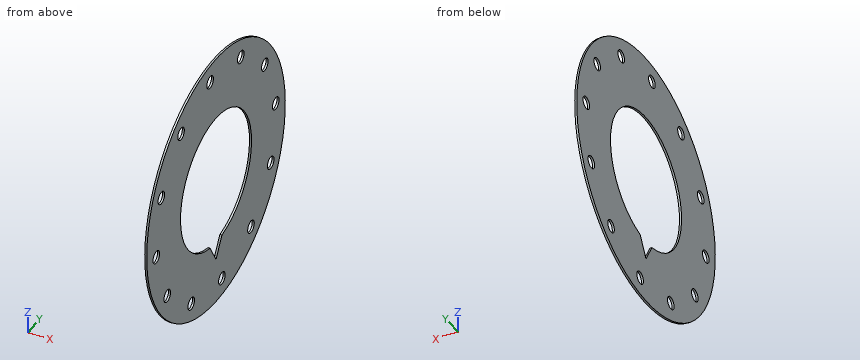
Autodesk Inventor part; units mm, degrees
ref_plane "SHAFT_MOUNTING_PLANE" through (9.525, 0, 0) normal (1, 0, 0) x (0, 1, 0)
ref_plane "UCSBasePlConstraintOrigin: YZ Plane" through (0, 0, 0) normal (0, 0, -1) x (0, 1, 0)
ref_plane "UCSBasePlConstraintOrigin: XZ Plane" through (0, 0, 0) normal (0, 1, 0) x (1, 0, 0)
ref_plane "BASE_PLATE_FACE" through (9.525, 0, 0) normal (1, 0, 0) x (0, 1, 0)
sketch "BASE_PLATE_SKETCH" plane through (9.525, 0, 0) normal (1, 0, 0) x (0, 0, -1)
  circle A0 centre (0, 0) radius 536.575 construction
  circle A1 centre (0, 0) radius 317.5
  line L0 (0, 536.575) -> (0, 536.575) construction
  circle A2 centre (0, 0) radius 619.125
  line L1 (0, 0) -> (-52.5935, -533.9912) construction
  line L2 (0, 0) -> (52.5935, -533.9912) construction
  line L3 (313.0592, 52.9167) -> (404.7136, 0)
  line L4 (404.7136, 0) -> (313.0592, -52.9167)
  line L5 (313.0592, -52.9167) -> (313.0592, 52.9167)
  line L6 (0, 0) -> (0, 536.575) construction
  line L7 (0, 0) -> (267.5578, 465.1081) construction
  point P0 (-619.125, 0)
  point P1 (619.125, 0)
  point P2 (0, 619.125)
  point P3 (0, -619.125)
  point P4 (0, 619.125)
  point P5 (619.125, 0)
  point P6 (0, -619.125)
  point P7 (-619.125, 0)
  point P8 (343.6107, 0)
  point P9 (313.0592, 0)
  point P10 (313.0592, -52.9167)
  dimension "GapSize" = 9.525
  dimension "SeamGap" = 0.0051
  dimension "Thickness" = 9.525
  dimension "BendRadius" = 9.525
  dimension "MinimumRemnant" = 19.05
  dimension "BendReliefDepth" = 4.7625
  dimension "BendReliefWidth" = 9.525
  dimension "CornerReliefSize" = 38.1
  dimension "JacobiRadiusSize" = 9.525
  dimension "TransitionRadius" = 9.525
  dimension "TEMPLATE_CENTER_HOLE_DIA" = 635
  dimension "NUMBER_OF_HOLES_IN_BOLT_PLATE" = 12
  dimension "BOLT_CIRCLE_DIA" = 1073.15
  dimension "TEMPLATE_DIA" = 1238.25
  dimension "PARENT_HOLE_ANG_L" = 5.625
  dimension "PARENT_HOLE_ANG_R" = 5.625
  dimension "NOTCH_LEG" = 105.8333
  dimension "d297" = 105.8333
  dimension "LEADER_PLACE_A_ANG" = 29.91
extrude "BASE_PLATE_BODY" add sketch "BASE_PLATE_SKETCH" against normal up to surface (9.525 mm away) contours A1 L3 L4 | A2
ref_plane "SHAFT_MOUNTING_PLANE" through (9.525, 0, 0) normal (1, 0, 0) x (0, 1, 0)
hole "PARENT_HOLE" at (9.525, -533.9912, -52.5935) direction (-1, 0, 0) diameter 58.7375 depth 9.525 tip angle 118
pattern_circular "BOLT_HOLES" count 12 over 360 about axis through (-10, 0, 0) along (1, 0, 0) of "PARENT_HOLE"
ref_plane "DimPlaneRight" through (0, 0, -619.125) normal (0, 0, 1) x (1, 0, 0)
ref_plane "DimPlaneLeft" through (0, 0, 619.125) normal (0, 0, 1) x (1, 0, 0)
ref_plane "DimPlaneTop" through (0, 619.125, 0) normal (0, 1, 0) x (-1, 0, 0)
ref_plane "DimPlaneBtm" through (0, -619.125, 0) normal (0, 1, 0) x (-1, 0, 0)
ref_plane "PLPointBngPltCenterHoleDia" through (0, 0, 0) normal (0, -0.866, 0.5) x (1, 0, 0)
extrude "V NOTCH CUT" cut sketch "BASE_PLATE_SKETCH" against normal through all contours A1 L3 L4
equation "\"BOLT_CIRCLE_DIA\" = INPUT_BOLT_CIRCLE_DIAMETER"
equation "\"INPUT_TEMPLATE_DIAMETER\" = 1238.25"
equation "\"INPUT_BOLT_HOLE_SIZE\" = 58.7375"
equation "\"INPUT_BOLT_CIRCLE_DIAMETER\" = 1073.15"
equation "\"INPUT_PARENT_HOLE_ANG_OFF_90_270\" = 5.625deg"
equation "\"SHAFT_B_DIST_AK_BOTTOM\" = 933.5008"
equation "\"SHAFT_B_DIST_AF_BOTTOM\" = 901.7"
equation "\"SHAFT_B_Thickness\" = 7.9502"
equation "\"INPUT_CENTER_HOLE_DIAMETER\" = 635"
equation "\"LEADER_PLACE_A\" = 68.5deg"
equation "\"TEMPLATE_RAD\" = 619.125"
properties part number "25-00000E_TEMPLATE_TOP" material "A572 GRADE 65"
Here's how the part is built. I have some questions about the finished solid (model axes, mm). Coordinates: 2 decimals unless noted, no trailing zeros. Write each loop counter-clockwise with the first axis right and the second up, starting at its lowest first coordinate (ties: lowest second). Pieces come first, ordered by that corner, then holes. Notation, with made-up numbers: (39.25, 84) - (60.25, 84) arc R20 cw to (60.25, 108) - close; hole circle Ø6 at (57, 43). An arc over 180 degrees is marked (long way). Use one line per item in the form item = value.
1) Suppose I cut it at C-C, the plane x = 6.25. Give the number of separate pieces and of enclosed holes in the cut face, plus the area to 3 significant figures.
Solved:
separate_pieces = 1
enclosed_holes = 13
area = 850,000 mm2
2) I need wall thicknesses on line 1 (Z direction, x = 2.5, y = -247); line 2 (Z direction, x = 6, y = 221.5); line 3 (Y direction, x = 3.75, z = 0) (3 decimals). Which ranges of each line are inside material? Lowest first, please.
Solved:
line_1 = -567.72 to -503.23, -474.27 to -199.49, 199.49 to 567.72
line_2 = -578.15 to -227.47, 227.47 to 459.38, 518.12 to 578.15
line_3 = -619.125 to -317.5, 317.5 to 619.125
3) Suppose I cut it at B-B, the plane z = 298. Write out the boundary of the cut face in (x, y) (3 decimals).
Solved:
outline = (0, -542.689) - (9.525, -542.689) - (9.525, -109.555) - (0, -109.555) - close; (0, 109.555) - (9.525, 109.555) - (9.525, 410.638) - (0, 410.638) - close; (0, 461.668) - (9.525, 461.668) - (9.525, 542.689) - (0, 542.689) - close
4) Suppose I cut it at D-D, the plane z = -210.5. Write out the boundary of the cut face in (x, y) (3 decimals).
Solved:
outline = (0, -582.242) - (9.525, -582.242) - (9.525, -237.689) - (0, -237.689) - close; (0, 237.689) - (9.525, 237.689) - (9.525, 461.495) - (0, 461.495) - close; (0, 515.998) - (9.525, 515.998) - (9.525, 582.242) - (0, 582.242) - close
5) Suppose I cut it at A-A, the plane z = 0. Write out the boundary of the cut face in (x, y) (3 decimals), plus the area to 3 significant figures.
Solved:
outline = (0, -619.125) - (9.525, -619.125) - (9.525, -317.5) - (0, -317.5) - close; (0, 317.5) - (9.525, 317.5) - (9.525, 619.125) - (0, 619.125) - close
area = 5,750 mm2
6) I'm going to push flat-ended pins straight in: P1, Ø1, axis at x = 2, y = -357.5, coming from the -Z side; P2, Ø5, axis at x = 7.5, y = -151.5, coming from the +Z side; P3, Ø1.5, axis at x = 4, z = 105, coming from the -Y side. Where does each tip first touch, or does it pass through?
Solved:
P1 = -505.83
P2 = 600.93
P3 = -610.28
